Input: dimensioned drawing with shaded views. Units: mm. Origin: part minimum x, y, z. Coordinates: 2 decimals unless noted, no trailing zeros. Loops run counter-clockwise (first coordinate to the right, second up) from the corner with the lowest first, then second, coordinate; pieces in that order, holes last. Notation, with made-up numbers: (80.5, 51.5) - (126.5, 51.5) arc R20 cw to (126.5, 69.5) - close; hole circle Ø6 at (-25, 6). An arc over 180 degrees is marked (long way). Use one line per item in the form item = value. Start each with the question number.
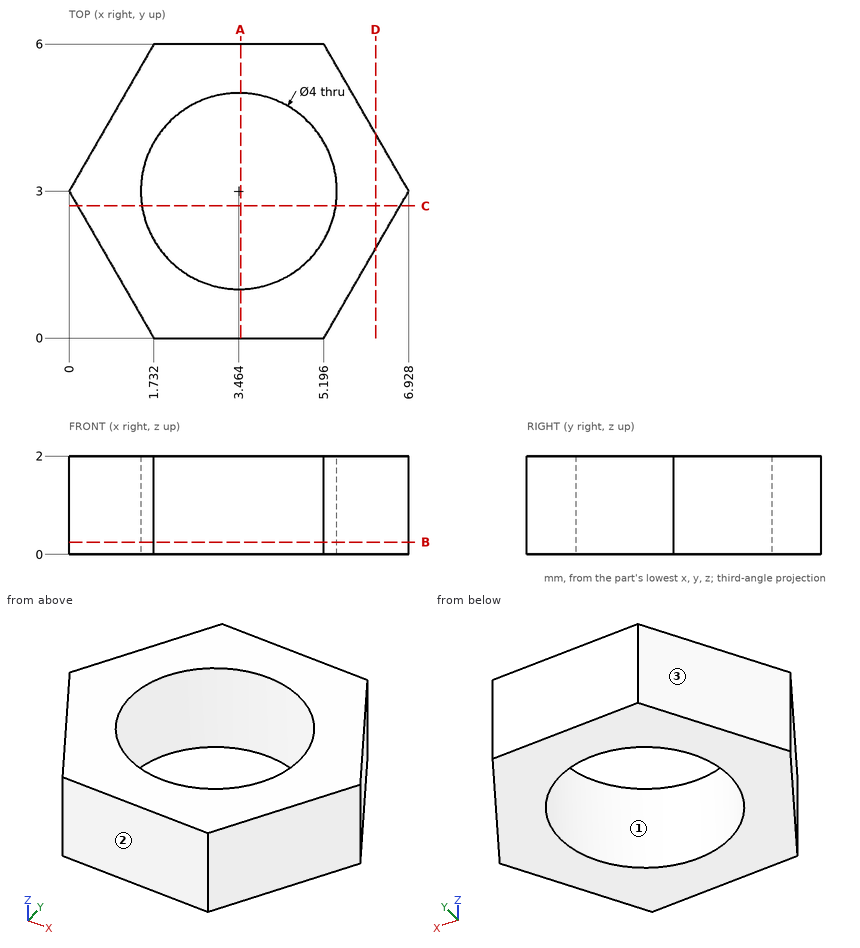
(1) Contact query for a flat-ended pin moving along its axis: pin 1 (3.5 mm diameter, centred on x = 3.46, y = 3, fed in from -Z). Output: stop coordinate, or through.
(2) Cut plane B-B, the plane z = 0.25. Output: boundary loops of the cut face in (x, y), plus the area to 3 significant figures.
(3) Mould query, pull axis Y, two halves, no side actions, for the marked faces 1, 2 and 3. Classes: +Y half, -Y half, draft (parallel to the pull), parting line (faces both ways), or undercut.
(4) Cut plane C-C, the plane y = 2.7. Output: boundary loops of the cut face in (x, z) (1 decimal).
(5) Cut plane D-D, the plane x = 6.25. Output: boundary loops of the cut face in (y, z) (1 decimal), plus the area to 3 significant figures.
(6) Material intervals for line 1 (Y direction, x = 3.5, z = 0.8); line 2 (X direction, y = 3.6, z = 0.6); line 3 (X direction, y = 1.75, z = 1.55) (1 decimal), sorted ascending.
(7) Cut plane A-A, the plane x = 3.5. Output: boundary loops of the cut face in (y, z).
Recorded:
q1.pin_1 = through
q2.outline = (0, 3) - (1.73, 0) - (5.2, 0) - (6.93, 3) - (5.2, 6) - (1.73, 6) - close; hole circle Ø4 at (3.46, 3)
q2.area = 18.6 mm²
q3.face_1 = undercut
q3.face_2 = -Y half
q3.face_3 = +Y half
q4.outline = (0.2, 0) - (1.5, 0) - (1.5, 2) - (0.2, 2) - close; (5.4, 0) - (6.8, 0) - (6.8, 2) - (5.4, 2) - close
q5.outline = (1.8, 0) - (4.2, 0) - (4.2, 2) - (1.8, 2) - close
q5.area = 4.70 mm²
q6.line_1 = 0 to 1, 5 to 6
q6.line_2 = 0.35 to 1.56, 5.37 to 6.58
q6.line_3 = 0.7 to 1.9, 5 to 6.2
q7.outline = (0, 0) - (1, 0) - (1, 2) - (0, 2) - close; (5, 0) - (6, 0) - (6, 2) - (5, 2) - close
